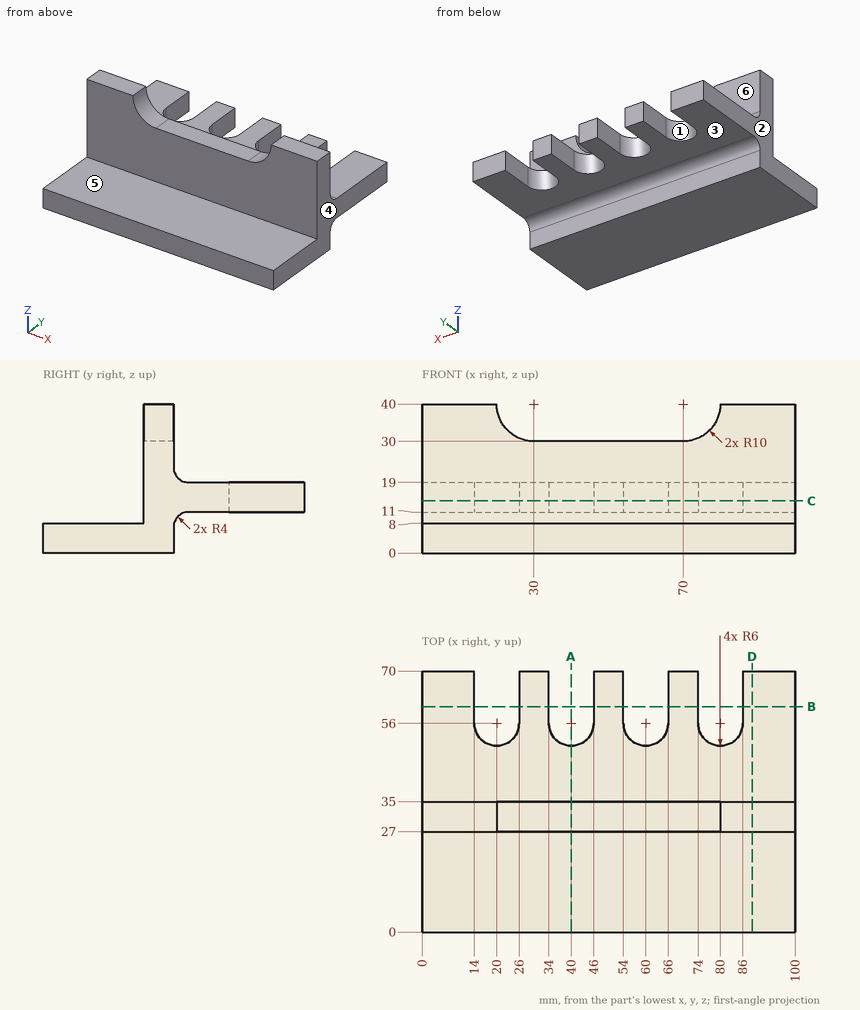
For this review, use the dimensioned drawing (mm, ordinates from the lowest corner) and the shaded views. A direction names the side the tool comes from. Give positions to 0.01 mm unless a question says otherwise; leave off trailing zeros. Order: outer loops, then holes, each group sorted by start corner. A loop starts at its lowest first (then second) coordinate and runs counter-clockwise, first axis right, second up. Notation, with made-up numbers: (4.5, 87.5) -> (50.5, 87.5) arc R24 cw to (50.5, 115.5) -> close; hole circle Ø9 at (33, -18). An arc over 180 degrees is marked (long way). Write item = value, one per line. Start each with the question number.
(1) Take a section at C-C (z = 14). Write out the cut boundary in (x, y), plus the area to 3 significant figures.
(2) Take a section at B-B (y = 60.5). Write out the cut boundary in (x, z).
(3) For pin 1 Ø7.5 at (x, z) = (25, 2.5) entering from +Y; pin 2 Ø4 at (x, y) = (59, 32) entering from +Z; pin 3 Ø8 at (x, y) = (58.5, 53) entering from +Z; pin 4 Ø4 at (x, y) = (16.5, 58.5) entering from -Z, all flat-tipped, find the tip position at first contact; note any pin that passes through.
(4) Take a section at D-D (x = 88.5). Write out the cut boundary in (y, z).
(5) Tool access review of the marked faces 4, 5 and 6: name each direction out of +Z, -Z, +X, -X, +Y, -Y from which nothing blocks a thin tool from reaching the whole face with its end or side.
(6) For L1, parallel to X at y = 61, z = 11.5; L2, parallel to X at y = 50.5, z = 16; L3, parallel to Z at x = 67, y = 57, list the stretches that pass through material, from the lowest coordinate up. Write a range as from..to.
(7) Take a section at A-A (x = 40). Write out the cut boundary in (y, z), plus the area to 3 significant figures.
(8) Draft analysis for pull direction X (two halves, no side actions). For the marked faces 1, 2 and 3, state which applies: +X half, -X half, draft (parallel to the pull), parting line (faces both ways), or undercut.
Returned:
q1.outline = (0, 27) -> (100, 27) -> (100, 70) -> (86, 70) -> (86, 56) arc R6 cw to (74, 56) -> (74, 70) -> (66, 70) -> (66, 56) arc R6 cw to (54, 56) -> (54, 70) -> (46, 70) -> (46, 56) arc R6 cw to (34, 56) -> (34, 70) -> (26, 70) -> (26, 56) arc R6 cw to (14, 56) -> (14, 70) -> (0, 70) -> close
q1.area = 3,400 mm²
q2.outline = (0, 11) -> (14, 11) -> (14, 19) -> (0, 19) -> close; (26, 11) -> (34, 11) -> (34, 19) -> (26, 19) -> close; (46, 11) -> (54, 11) -> (54, 19) -> (46, 19) -> close; (66, 11) -> (74, 11) -> (74, 19) -> (66, 19) -> close; (86, 11) -> (100, 11) -> (100, 19) -> (86, 19) -> close
q3.pin_1 = 35
q3.pin_2 = 30
q3.pin_3 = 19
q3.pin_4 = through
q4.outline = (0, 0) -> (35, 0) -> (35, 7) arc R4 cw to (39, 11) -> (70, 11) -> (70, 19) -> (39, 19) arc R4 cw to (35, 23) -> (35, 40) -> (27, 40) -> (27, 8) -> (0, 8) -> close
q5.face_4 = +Z, -Z, +X, +Y, -Y
q5.face_5 = +Z, +X, -X, -Y
q5.face_6 = +Z, +X, -X, +Y
q6.L1 = 0..14, 26..34, 46..54, 66..74, 86..100
q6.L2 = 0..17.6, 22.4..37.6, 42.4..57.6, 62.4..77.6, 82.4..100
q6.L3 = 11..19
q7.outline = (0, 0) -> (35, 0) -> (35, 7) arc R4 cw to (39, 11) -> (50, 11) -> (50, 19) -> (39, 19) arc R4 cw to (35, 23) -> (35, 30) -> (27, 30) -> (27, 8) -> (0, 8) -> close
q7.area = 583 mm²
q8.face_1 = undercut
q8.face_2 = -X half
q8.face_3 = draft
